from build123d import *

# Parameters (mm, degrees)
SKETCH1_W           = 24.0664
SKETCH1_H           = 28.5
BOSS_EXTRUDE1_DEPTH = 14.5651
CUT_EXTRUDE1_DEPTH  = 35.193421008
CUT_EXTRUDE2_DEPTH  = 2


with BuildPart() as part:
    # Sketch1 → Boss-Extrude1 (new body)
    with BuildSketch(Plane(origin=(0, 0, 0), x_dir=(0, 1, 0), z_dir=(0, 0, 1))):
        Rectangle(SKETCH1_W, SKETCH1_H)
    extrude(amount=BOSS_EXTRUDE1_DEPTH)

    # Sketch2 → Cut-Extrude1 (cut, through all)
    with BuildSketch(Plane.YZ.offset(14.25)):
        Polygon((-10.0332, 12.8151), (10.0332, 12.8151), (10.0332, 1.75), (8.5, 1.75), (8.5, 0), (-8.5, 0), (-8.5, 1.75), (-10.0332, 1.75), align=None)
    extrude(amount=-CUT_EXTRUDE1_DEPTH, mode=Mode.SUBTRACT)

    # Sketch4 → Cut-Extrude2 (cut)
    with BuildSketch(Plane.YZ.offset(14.25)):
        Polygon((10.0332, 1.75), (10.5332, 1.75), (10.5332, 0), (8.5, 0), (8.5, 1.75), align=None)
        Polygon((-10.5332, 0), (-10.5332, 1.75), (-10.0332, 1.75), (-8.5, 1.75), (-8.5, 0), align=None)
    extrude(amount=-CUT_EXTRUDE2_DEPTH, mode=Mode.SUBTRACT)


solid = part.part
Here's how the part is built. I have some questions about the finished solid (model axes, mm). A direction names the side the tool comes from. Round coordinates to 2 decimals unless told otherwise and drop trailing zeros. Loops run counter-clockwise (first coordinate to the right, second up) from the corner with the lowest first, then second, coordinate; pieces in that order, holes last.
1. We'd pull the mould along Z, two halves only. Please class faces 1 (the face through (0, 0, 14.565)), 2 (the face through (0, 10.033, 7)), 3 (the face through (13, -10.533, 1)): +Z half, -Z half, draft (parallel to the pull), parting line (faces both ways), or undercut.
Answer list:
face 1: +Z half
face 2: undercut
face 3: draft
2. If we section it at B-B on x = 2.25: Write out the boundary of the cut face in (y, z), plus the area to 3 significant figures.
Answer list:
outline: (-12.03, 0) - (-8.5, 0) - (-8.5, 1.75) - (-10.03, 1.75) - (-10.03, 12.82) - (10.03, 12.82) - (10.03, 1.75) - (8.5, 1.75) - (8.5, 0) - (12.03, 0) - (12.03, 14.57) - (-12.03, 14.57) - close
area: 98.7 mm2
3. If we section it at C-C on y = 1.25: Write out the boundary of the cut face in (x, z), plus the area to 3 significant figures.
Answer list:
outline: (-14.25, 12.82) - (14.25, 12.82) - (14.25, 14.57) - (-14.25, 14.57) - close
area: 49.9 mm2
4. Which directions (+Z, -Z, +X, -X, +Y, -Y) give clear straight access to the entire face, cutting with the end or side of a thin tool? Please do faces 4 (the face through (-1, -8.5, 1)), 5 (the face through (-14.25, 0, 13)), 6 (the face through (0, 10, 0)), 7 (the face through (-1, 9, 1.75)), 8 (the face through (12.25, 10, 1)).
Answer list:
face 4: -Z, +X, -X
face 5: +Z, -Z, -X, +Y, -Y
face 6: -Z, +X, -X, +Y, -Y
face 7: +X, -X
face 8: -Z, +X
5. If I drill on line 1 along Y through (x, z) = (-10, 3.5); line 2 along Y through (x, z) = (10, 0.75); line 3 along Z through (x, y) = (-4.5, 0), over which ranges is the centre line in solid material (lowest first)?
Answer list:
line 1: y = -12.03 to -10.03, 10.03 to 12.03
line 2: y = -12.03 to -8.5, 8.5 to 12.03
line 3: z = 12.82 to 14.57
6. For P1, Ø6, axis at x = -6, y = 0.5, coming from the -Z side; P2, Ø0.5, axis at y = 10, z = 1, coming from the +X side; P3, Ø10, axis at x = 5, y = -8.5, coming from the -Z side, each with a flat end and sliding along its axis, tell me the tip position at first contact or that it passes through.
Answer list:
P1: stops at z = 12.82
P2: stops at x = 12.25
P3: stops at z = 0
7. If we section it at A-A on z = 6.75: Write out the boundary of the cut face in (x, y), plus the area to 3 significant figures.
Answer list:
outline: (-14.25, -12.03) - (14.25, -12.03) - (14.25, -10.03) - (-14.25, -10.03) - close; (-14.25, 10.03) - (14.25, 10.03) - (14.25, 12.03) - (-14.25, 12.03) - close
area: 114 mm2
